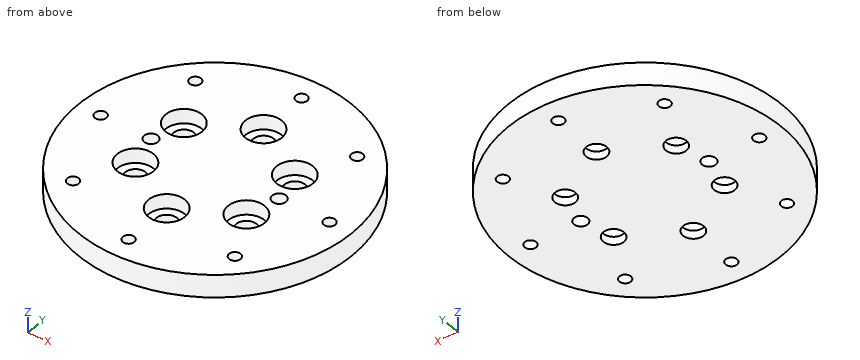
```python
from build123d import *

# Parameters (mm, degrees)
SKETCH1_R                                            = 30
BOSS_EXTRUDE1_DEPTH                                  = 5
CBORE_FOR_M4_HEX_SOCKET_THIN_HEAD_CAP_SC_D           = 4.5
CBORE_FOR_M4_HEX_SOCKET_THIN_HEAD_CAP_SC_CBORE_D     = 8
CBORE_FOR_M4_HEX_SOCKET_THIN_HEAD_CAP_SC_CBORE_DEPTH = 3.2
F_3_0MM_DOWEL_HOLE1_OUTLINE_R                        = 1.5
F_3_0MM_DOWEL_HOLE1_DEPTH                            = 5
TAP_DRILL_FOR_M3_TAP1_D                              = 2.5


# Read off the part's stored shape, not the designer's step: Ø3.0mm Dowel Hole1
with BuildPart() as part:
    # Sketch1 → Boss-Extrude1 (new body)
    with BuildSketch(Plane.XY):
        Circle(SKETCH1_R)
    extrude(amount=BOSS_EXTRUDE1_DEPTH)

    # CBORE for M4 Hex Socket Thin Head Cap Screw1 (through all)
    with Locations(Plane.XY.offset(5)):
        with Locations((-12.124355653, 7), (0, 14), (12.124355653, 7), (12.124355653, -7), (0, -14), (-12.124355653, -7)):
            CounterBoreHole(CBORE_FOR_M4_HEX_SOCKET_THIN_HEAD_CAP_SC_D / 2, CBORE_FOR_M4_HEX_SOCKET_THIN_HEAD_CAP_SC_CBORE_D / 2, CBORE_FOR_M4_HEX_SOCKET_THIN_HEAD_CAP_SC_CBORE_DEPTH)

    # Ø3.0mm Dowel Hole1 outline → Ø3.0mm Dowel Hole1 (cut)
    with BuildSketch(Plane.XY):
        with Locations((14, 0)):
            Circle(F_3_0MM_DOWEL_HOLE1_OUTLINE_R)
        with Locations((-14, 0)):
            Circle(F_3_0MM_DOWEL_HOLE1_OUTLINE_R)
    extrude(amount=F_3_0MM_DOWEL_HOLE1_DEPTH, mode=Mode.SUBTRACT)

    # Tap Drill for M3 Tap1 (through all)
    with Locations(Plane.XY.offset(5)):
        with Locations((-17.67766953, 17.67766953), (0, 25), (17.67766953, 17.67766953), (25, 0), (17.67766953, -17.67766953), (0, -25), (-17.67766953, -17.67766953), (-25, 0)):
            Hole(TAP_DRILL_FOR_M3_TAP1_D / 2)


solid = part.part
```
Could you check a few things on this model? Use its own coordinates, in mm. Give positions to 0.01 mm unless a question says otherwise; leave off trailing zeros. Order: outer loops, then holes, each group sorted by start corner. A loop starts at its lowest first (then second) coordinate and runs counter-clockwise, first axis right, second up.
Q1. If I drill on line 1 along Y through (x, z) = (0, 1.05); line 2 along Y through (x, z) = (1.5, 0.85); line 3 along Y through (x, z) = (-14, 3.35), over which ranges is the centre line in solid material (lowest first)?
Q2. I'm going to push flat-ended pins straight in: P1, Ø1.5, axis at y = -3, z = 3.5, coming from the -X side; P2, Ø4, axis at x = -13, y = 6, coming from the +Z side; P3, Ø1.5, axis at y = -5, z = 1.5, coming from the +X side. Where does each tip first touch, or does it pass through?
Q3. Suppose I cut it at C-C, the plane z = 1.1. Count the separate pieces of the cut face and the enclosed holes in it, and give its area (3 significant figures).
Q4. Suppose I cut it at A-A, the plane x = 0. Write out the boundary of the cut face in (y, z).
Q5. Suppose I cut it at D-D, the plane x = 25. Write out the boundary of the cut face in (y, z), and give its area (3 significant figures).
Q6. Suppose I cut it at B-B, the plane y = 0. Write out the boundary of the cut face in (x, z), and give its area (3 significant figures).
Solution:
1. line 1: y = -30 to -26.25, -23.75 to -16.25, -11.75 to 11.75, 16.25 to 23.75, 26.25 to 30
1. line 2: y = -29.96 to -15.68, -12.32 to 12.32, 15.68 to 29.96
1. line 3: y = -26.53 to -10.53, -3.47 to -1.5, 1.5 to 3.47, 10.53 to 26.53
2. P1: stops at x = -29.92
2. P2: stops at z = 1.8
2. P3: stops at x = 29.7
3. separate pieces: 1
3. enclosed holes: 16
3. area: 2,680 mm2
4. outline: (-30, 0) - (-26.25, 0) - (-26.25, 5) - (-30, 5) - close; (-23.75, 0) - (-16.25, 0) - (-16.25, 1.8) - (-18, 1.8) - (-18, 5) - (-23.75, 5) - close; (-11.75, 0) - (11.75, 0) - (11.75, 1.8) - (10, 1.8) - (10, 5) - (-10, 5) - (-10, 1.8) - (-11.75, 1.8) - close; (16.25, 0) - (23.75, 0) - (23.75, 5) - (18, 5) - (18, 1.8) - (16.25, 1.8) - close; (26.25, 0) - (30, 0) - (30, 5) - (26.25, 5) - close
5. outline: (-16.58, 0) - (-1.25, 0) - (-1.25, 5) - (-16.58, 5) - close; (1.25, 0) - (16.58, 0) - (16.58, 5) - (1.25, 5) - close
5. area: 153 mm2
6. outline: (-30, 0) - (-26.25, 0) - (-26.25, 5) - (-30, 5) - close; (-23.75, 0) - (-15.5, 0) - (-15.5, 5) - (-23.75, 5) - close; (-12.5, 0) - (12.5, 0) - (12.5, 5) - (-12.5, 5) - close; (15.5, 0) - (23.75, 0) - (23.75, 5) - (15.5, 5) - close; (26.25, 0) - (30, 0) - (30, 5) - (26.25, 5) - close
6. area: 245 mm2
